Can you work these out from the drawing? Everything is in mm from the part's minimum corner. A direction names the side the tool comes from. Round coordinates to 2 decimals unless told otherwise and drop trailing zeros. Write each loop counter-clockwise with the first axis right and the second up, starting at its lowest first coordinate (ties: lowest second). Pieces come first, ordered by that corner, then holes. Notation, with made-up numbers: (9.25, 29.5) -> (56.25, 29.5) arc R21 cw to (56.25, 45.5) -> close; hole circle Ø8 at (58.5, 84.25). An arc over 180 degrees is marked (long way). One line per question, with ' | ' between items. Start each with the question number.
1. Imagine slicing it at B-B, the plane x = 4.5. List the corners of the cut face in (y, z) for me.
2. Imagine slicing it at C-C, the plane y = 23.75. List the corners of the cut face in (x, z) for me, and give its area (3 significant figures).
3. Thinking about a two-plate mould opening in X: for the marked faces 1, 2, 3 and 4, which applies, released by +X, released by -X, zero draft, split by the parting line, or undercut?
4. If I drill on line 1 along Z through (x, y) = (4.5, 1.85); line 2 along Z through (x, y) = (14.5, 25.8); line 3 along Y through (x, z) = (14.5, 3.25), over which ranges is the centre line in solid material (lowest first)? Write a range as [from, to].
5. Imagine slicing it at A-A, the plane z = 5. List the corners of the cut face in (x, y) for me.
6. For pin 1 Ø3 at (y, z) = (17, 3) entering from -X; pin 2 Ø1.5 at (x, z) = (18.5, 9) entering from -Y; pin 3 Ø2.5 at (x, z) = (14.5, 5) entering from +Y, each with a flat end and sliding along its axis, tell me the tip position at first contact or that it passes through.
7. Imagine slicing it at D-D, the plane x = 14.5. List the corners of the cut face in (y, z) for me, and give its area (4 significant figures).
8. For the marked faces 5, 6 and 7, which set-ups out of +Z, -Z, +X, -X, +Y, -Y let a thin tool reach every point of the face, with its end or its side?
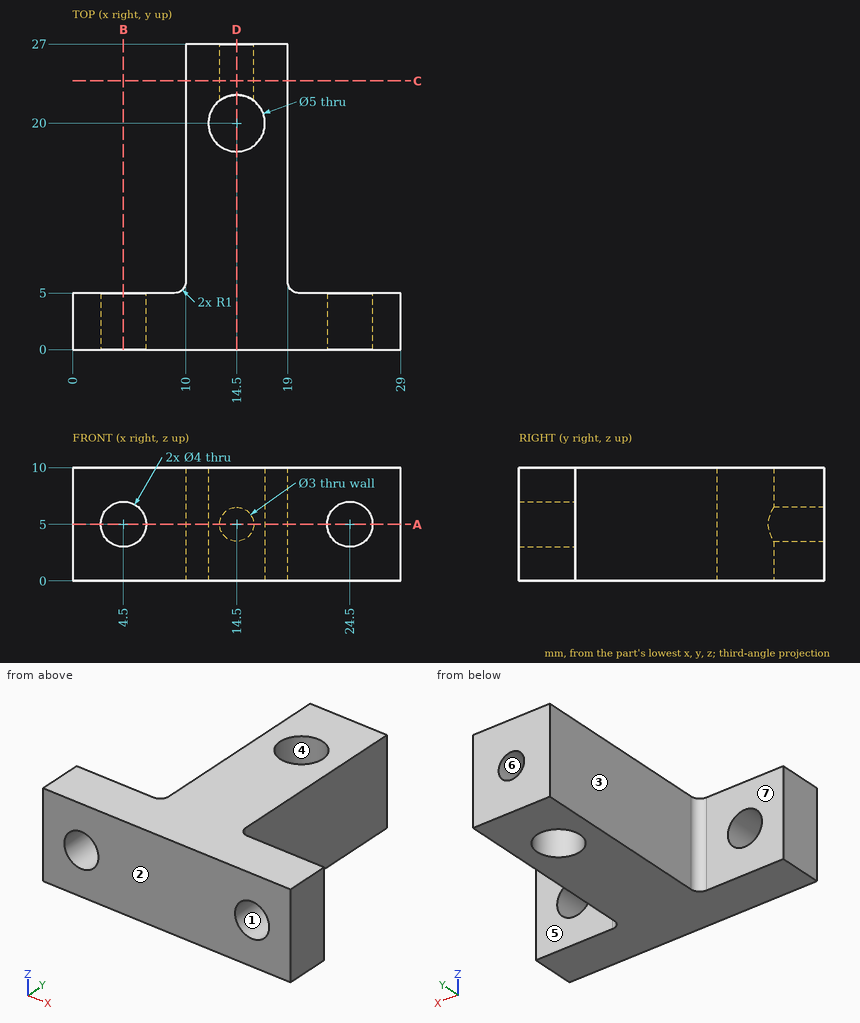
Geometry results:
1) outline: (0, 0) -> (5, 0) -> (5, 3) -> (0, 3) -> close; (0, 7) -> (5, 7) -> (5, 10) -> (0, 10) -> close
2) outline: (10, 0) -> (19, 0) -> (19, 10) -> (10, 10) -> close; hole circle Ø3 at (14.5, 5) | area: 82.9 mm2
3) face 1: undercut | face 2: zero draft | face 3: released by -X | face 4: undercut
4) line 1: z = [0, 3], [7, 10] | line 2: z = [0, 3.5], [6.5, 10] | line 3: y = [0, 17.5], [22.5, 27]
5) outline: (0, 0) -> (2.5, 0) -> (2.5, 5) -> (0, 5) -> close; (6.5, 0) -> (22.5, 0) -> (22.5, 5) -> (20, 5) arc R1 cw to (19, 6) -> (19, 27) -> (16, 27) -> (16, 22) arc R2.5 cw (long way) to (13, 22) -> (13, 27) -> (10, 27) -> (10, 6) arc R1 cw to (9, 5) -> (6.5, 5) -> close; (26.5, 0) -> (29, 0) -> (29, 5) -> (26.5, 5) -> close
6) pin 1: stops at x = 10 | pin 2: stops at y = 0 | pin 3: stops at y = 17.83
7) outline: (0, 0) -> (17.5, 0) -> (17.5, 10) -> (0, 10) -> close; (22.5, 0) -> (27, 0) -> (27, 3.5) -> (22.5, 3.5) -> close; (22.5, 6.5) -> (27, 6.5) -> (27, 10) -> (22.5, 10) -> close | area: 206.5 mm2
8) face 5: +Z, -Z, +X, +Y | face 6: +Y | face 7: +Z, -Z, -X, +Y
